Autodesk Inventor part; units mm, degrees
ref_plane "YZ Plane" through (0, 0, 0) normal (1, 0, 0) x (0, 1, 0)
ref_plane "XZ Plane" through (0, 0, 0) normal (0, 1, 0) x (-1, 0, 0)
ref_plane "XY Plane" through (0, 0, 0) normal (0, 0, 1) x (1, 0, 0)
sketch "Sketch4" plane through (0, 0, 0) normal (0, 1, 0) x (-1, 0, 0)
  line L0 (0, 0) -> (25, 0)
  line L1 (25, 0) -> (25, -27)
  line L2 (25, -27) -> (0, -27)
  line L3 (0, -27) -> (0, 0)
  line L4 (25, 0) -> (18, 0)
  circle A0 centre (18, -6) radius 2.5
  circle A1 centre (18, -21) radius 2.5
  dimension "d35" = 25
  dimension "d36" = 27
  dimension "d39" = 5
  dimension "d41" = 5
extrude "Extrusion4" add sketch "Sketch4" along normal blind 38
sketch "Sketch5" plane through (0, 38, 0) normal (0, 1, 0) x (1, 0, 0)
  line L0 (0, 0) -> (0, 27)
  line L1 (0, 0) -> (0, 27)
  line L2 (0, 27) -> (0, 13.5)
  line L3 (0, 13.5) -> (-10, 13.5)
  circle A0 centre (-10, 13.5) radius 4
  dimension "d44" = 10
  dimension "d51" = 8
extrude "Extrusion5" add sketch "Sketch5" along normal blind 20
chamfer "Chamfer2" distance 2 angle 45 4 edges at (-25, 19, 0) (-25, 19, -27) (0, 19, -27) (0, 19, 0)
properties part number "pneumaticActuator"
Check sheet for the modelled part. Datum: model origin and axes. Units: mm. A direction names the side the tool comes from. Give positions to 0.01 mm unless a question says otherwise; leave off trailing zeros. Order: outer loops, then holes, each group sorted by start corner. A loop starts at its lowest first (then second) coordinate and runs counter-clockwise, first axis right, second up. Notation, with made-up numbers: (17, 63.25) -> (40, 63.25) arc R26 cw to (40, 92.25) -> close; hole circle Ø7 at (39, 60). An arc over 180 degrees is marked (long way). Use CSV: the item, a comma, the result in double quotes. Start each with the question number.
1) Material ranges on line 1 (Z direction, x = -18, y = 26); line 2 (Z direction, x = -15.75, y = 16); line 3 (Y direction, x = -12, z = -2.5), recorded low to high. Write a range as from..to.
2) Mould release check, pull along X, two halves, no side actions. Record for faces 1 (the face through (-16.16, 18.73, -22.69)), 2 (the face through (-24, 19, -1)), 3 (the face through (-10, 58, -14)): released by +X, released by -X, zero draft, split by the parting line, or undercut.
3) Sectioned sample at C-C, the plane y = 30. Record the boundary of the cut face in (x, z), plus the area to 3 significant figures.
4) Sectioned sample at B-B, the plane x = -18. Record the boundary of the cut face in (y, z), plus the area to 3 significant figures.
5) Sectioned sample at D-D, the plane x = -10. Record the boundary of the cut face in (y, z), plus the area to 3 significant figures.
6) Sectioned sample at A-A, the plane z = -21. Record the boundary of the cut face in (x, y).
7) Go/stop test with flat-tipped pins: P1, Ø8, axis at y = 43.5, z = -13.5, coming from the +X side; P2, Ø10, axis at x = -15.5, y = 46, coming from the -Z side; P3, Ø8, axis at x = -18, z = -23.5, coming from the +Y side. Record where each tip stops, or that it passes through.
8) Set-up check for faces 4 (the face through (-13.996, 47.86, -13.324)), 5 (the face through (-12, 19, 0)): record each of +Z, -Z, +X, -X, +Y, -Y from which the full face is reachable in a straight line by a thin tool's end or side.
Recorded:
1,line 1,"-27..-23.5, -18.5..-8.5, -3.5..0"
1,line 2,"-27..-22.09, -19.91..-7.09, -4.91..0"
1,line 3,"0..38"
2,face 1,"undercut"
2,face 2,"released by -X"
2,face 3,"zero draft"
3,outline,"(-25, -25) -> (-23, -27) -> (-2, -27) -> (0, -25) -> (0, -2) -> (-2, 0) -> (-23, 0) -> (-25, -2) -> close; hole circle Ø5 at (-18, -21); hole circle Ø5 at (-18, -6)"
3,area,"628 mm2"
4,outline,"(0, -27) -> (38, -27) -> (38, -23.5) -> (0, -23.5) -> close; (0, -18.5) -> (38, -18.5) -> (38, -8.5) -> (0, -8.5) -> close; (0, -3.5) -> (38, -3.5) -> (38, 0) -> (0, 0) -> close"
4,area,"646 mm2"
5,outline,"(0, -27) -> (38, -27) -> (38, -17.5) -> (58, -17.5) -> (58, -9.5) -> (38, -9.5) -> (38, 0) -> (0, 0) -> close"
5,area,"1,190 mm2"
6,outline,"(-25, 0) -> (-20.5, 0) -> (-20.5, 38) -> (-25, 38) -> close; (-15.5, 0) -> (0, 0) -> (0, 38) -> (-15.5, 38) -> close"
7,P1,"x = -6"
7,P2,"z = -17.47"
7,P3,"y = 38"
8,face 4,"+Y"
8,face 5,"+Z, +X, -X, +Y, -Y"
